Geometry: final body of the model. Coordinates: model frame, mm. A direction names the side the tool comes from. Give positions to 0.01 mm unless a question says otherwise; leave off trailing zeros. Loops run counter-clockwise (first coordinate to the right, second up) from the corner with the lowest first, then second, coordinate; pieces in that order, holes last.
from build123d import *

# Parameters (mm, degrees)
SZKIC1_R                    = 50
SZKIC1_R_2                  = 2
DODANIE_WYCI_GNI_CIE1_DEPTH = 10
SZKIC2_R                    = 21.25
SZKIC2_R_2                  = 1.75
SZKIC2_R_3                  = 10
WYTNIJ_WYCI_GNI_CIE3_DEPTH  = 5
SZKIC2_8_R                  = 1.75
SZKIC2_8_R_2                = 10
WYTNIJ_WYCI_GNI_CIE6_DEPTH  = 11


with BuildPart() as part:
    # Szkic1 → Dodanie-wyci_gni_cie1 (new body)
    with BuildSketch(Plane(origin=(0, 0, 0), x_dir=(1, 0, 0), z_dir=(0, 1, 0))):
        Circle(SZKIC1_R)
        with BuildLine():
            ThreePointArc((-28.838834765, 32.374368671), (-32.374368671, 32.374368671), (-32.374368671, 28.838834765))
            Line((-32.374368671, 28.838834765), (-21.767766953, 18.232233047))
            ThreePointArc((-21.767766953, 18.232233047), (-18.232233047, 18.232233047), (-18.232233047, 21.767766953))
            Line((-18.232233047, 21.767766953), (-28.838834765, 32.374368671))
        make_face(mode=Mode.SUBTRACT)
        with BuildLine():
            ThreePointArc((-32.374368671, -28.838834765), (-32.374368671, -32.374368671), (-28.838834765, -32.374368671))
            Line((-28.838834765, -32.374368671), (-18.232233047, -21.767766953))
            ThreePointArc((-18.232233047, -21.767766953), (-18.232233047, -18.232233047), (-21.767766953, -18.232233047))
            Line((-21.767766953, -18.232233047), (-32.374368671, -28.838834765))
        make_face(mode=Mode.SUBTRACT)
        with BuildLine():
            ThreePointArc((28.838834765, -32.374368671), (32.374368671, -32.374368671), (32.374368671, -28.838834765))
            Line((32.374368671, -28.838834765), (21.767766953, -18.232233047))
            ThreePointArc((21.767766953, -18.232233047), (18.232233047, -18.232233047), (18.232233047, -21.767766953))
            Line((18.232233047, -21.767766953), (28.838834765, -32.374368671))
        make_face(mode=Mode.SUBTRACT)
        with BuildLine():
            ThreePointArc((32.374368671, 28.838834765), (32.374368671, 32.374368671), (28.838834765, 32.374368671))
            Line((28.838834765, 32.374368671), (18.232233047, 21.767766953))
            ThreePointArc((18.232233047, 21.767766953), (18.232233047, 18.232233047), (21.767766953, 18.232233047))
            Line((21.767766953, 18.232233047), (32.374368671, 28.838834765))
        make_face(mode=Mode.SUBTRACT)
        with BuildLine():
            ThreePointArc((-31.466251763, -48.436814511), (-25.799706685, -45.41900176), (-19.413503243, -46.077281732))
            ThreePointArc((-19.413503243, -46.077281732), (-35.355339059, -35.355339059), (-46.077281732, -19.413503243))
            ThreePointArc((-46.077281732, -19.413503243), (-45.41900176, -25.799706685), (-48.436814511, -31.466251763))
            ThreePointArc((-48.436814511, -31.466251763), (-48.436814511, -48.436814511), (-31.466251763, -48.436814511))
        make_face()
        with Locations((-39.951533137, -39.951533137)):
            Circle(SZKIC1_R_2, mode=Mode.SUBTRACT)
        with BuildLine():
            ThreePointArc((-46.077281732, 19.413503243), (-35.355339059, 35.355339059), (-19.413503243, 46.077281732))
            ThreePointArc((-19.413503243, 46.077281732), (-25.799706685, 45.41900176), (-31.466251763, 48.436814511))
            ThreePointArc((-31.466251763, 48.436814511), (-48.436814511, 48.436814511), (-48.436814511, 31.466251763))
            ThreePointArc((-48.436814511, 31.466251763), (-45.41900176, 25.799706685), (-46.077281732, 19.413503243))
        make_face()
        with Locations((-39.951533137, 39.951533137)):
            Circle(SZKIC1_R_2, mode=Mode.SUBTRACT)
        with BuildLine():
            ThreePointArc((19.413503243, 46.077281732), (35.355339059, 35.355339059), (46.077281732, 19.413503243))
            ThreePointArc((46.077281732, 19.413503243), (45.41900176, 25.799706685), (48.436814511, 31.466251763))
            ThreePointArc((48.436814511, 31.466251763), (48.436814511, 48.436814511), (31.466251763, 48.436814511))
            ThreePointArc((31.466251763, 48.436814511), (25.799706685, 45.41900176), (19.413503243, 46.077281732))
        make_face()
        with Locations((39.951533137, 39.951533137)):
            Circle(SZKIC1_R_2, mode=Mode.SUBTRACT)
        with BuildLine():
            ThreePointArc((48.436814511, -31.466251763), (45.41900176, -25.799706685), (46.077281732, -19.413503243))
            ThreePointArc((46.077281732, -19.413503243), (35.355339059, -35.355339059), (19.413503243, -46.077281732))
            ThreePointArc((19.413503243, -46.077281732), (25.799706685, -45.41900176), (31.466251763, -48.436814511))
            ThreePointArc((31.466251763, -48.436814511), (48.436814511, -48.436814511), (48.436814511, -31.466251763))
        make_face()
        with Locations((39.951533137, -39.951533137)):
            Circle(SZKIC1_R_2, mode=Mode.SUBTRACT)
    extrude(amount=DODANIE_WYCI_GNI_CIE1_DEPTH)

    # Szkic2 → Wytnij-wyci_gni_cie3 (cut)
    with BuildSketch(Plane.XZ):
        Circle(SZKIC2_R)
        with Locations((0, 14.5)):
            Circle(SZKIC2_R_2, mode=Mode.SUBTRACT)
        with Locations((12.558868355, -7.249133975)):
            Circle(SZKIC2_R_2, mode=Mode.SUBTRACT)
        with Locations((-12.555868355, -7.250866025)):
            Circle(SZKIC2_R_2, mode=Mode.SUBTRACT)
        Circle(SZKIC2_R_3, mode=Mode.SUBTRACT)
    extrude(amount=-WYTNIJ_WYCI_GNI_CIE3_DEPTH, mode=Mode.SUBTRACT)

    # Szkic2_8 → Wytnij-wyci_gni_cie6 (cut, through all)
    with BuildSketch(Plane.XZ):
        with Locations((0, 14.5)):
            Circle(SZKIC2_8_R)
        with Locations((12.558868355, -7.249133975)):
            Circle(SZKIC2_8_R)
        with Locations((-12.555868355, -7.250866025)):
            Circle(SZKIC2_8_R)
        Circle(SZKIC2_8_R_2)
    extrude(amount=-WYTNIJ_WYCI_GNI_CIE6_DEPTH, mode=Mode.SUBTRACT)


solid = part.part
Item 1: Section query B-B on x = -7. Return loops of the section in (y, z).
Values follow:
outline: (0, -49.51) - (10, -49.51) - (10, -7.14) - (5, -7.14) - (5, -20.06) - (0, -20.06) - close; (0, 20.06) - (5, 20.06) - (5, 7.14) - (10, 7.14) - (10, 49.51) - (0, 49.51) - close
Item 2: Pin query (flat end, axial travel): pin 1 (5 mm diameter, centred on x = 29, y = 1.5, fed in from -Z); pin 2 (5 mm diameter, centred on x = -39.95, z = -39.95, fed in from +Y); pin 3 (1 mm diameter, centred on y = 8.5, z = -24, fed in from +X); pin 4 (1 mm diameter, centred on y = 5.5, z = 25.5, fed in from +X). Return the tip coordinate at first contact, or that it passes through.
Values follow:
pin 1: stops at z = -48.47
pin 2: stops at y = 10
pin 3: stops at x = 45.24
pin 4: stops at x = 45.46
Item 3: Draft query along Z for faces 4 (the face through (0, 5, -50)), 5 (the face through (25.7, 4.9, 45.4)), 6 (the face through (-32.34, 4.93, -32.41)). Return one class per face: +Z half, -Z half, draft (parallel to the pull), parting line (faces both ways), or undercut.
Values follow:
face 4: -Z half
face 5: +Z half
face 6: undercut
Item 4: Section query C-C on z = 26. Return loops of the section in (x, y), plus the area to 3 significant figures.
Values follow:
outline: (-45.46, 0) - (-29.54, 0) - (-29.54, 10) - (-45.46, 10) - close; (-22.46, 0) - (22.46, 0) - (22.46, 10) - (-22.46, 10) - close; (29.54, 0) - (45.46, 0) - (45.46, 10) - (29.54, 10) - close
area: 768 mm2
Item 5: Section query A-A on z = 0. Return loops of the section in (x, y), plus the area to 4 significant figures.
Values follow:
outline: (-50, 0) - (-21.25, 0) - (-21.25, 5) - (-10, 5) - (-10, 10) - (-50, 10) - close; (10, 5) - (21.25, 5) - (21.25, 0) - (50, 0) - (50, 10) - (10, 10) - close
area: 687.5 mm2
Item 6: Set-up query: faces 1 (the face through (-23.61, 4.93, 27.145)), 2 (the face through (-25.889, 4.93, 45.437)), 3 (the face through (4.42, 5, -9.15)). Return all of +Z, -Z, +X, -X, +Y, -Y with unobstructed straight access to the full face (end or side cutting, diameter ignored); none if empty.
Values follow:
face 1: +Y, -Y
face 2: +Z, +Y, -Y
face 3: -Y
Item 7: Ray query, probe 1 along Z at (x, y) = (29.5, 2); probe 2 along X at (y, z) = (8, -31); probe 3 along Z at (x, y) = (0, 2.75). Return the intervals inside material, ascending.
Values follow:
probe 1: z = -46.88 to -32.85, -25.96 to 25.96, 32.85 to 46.88
probe 2: x = -48 to -33.08, -27.46 to 27.46, 33.08 to 48
probe 3: z = -50 to -21.25, 21.25 to 50
Item 8: Section query D-D on y = 7.75. Give the number of separate pieces and of enclosed holes in the cut face, plus the area to 3 significant figures.
Values follow:
separate pieces: 1
enclosed holes: 12
area: 8,750 mm2
